For this review, take the finished solid that the model builds, in its own axes (mm). Coordinates: 2 decimals unless noted, no trailing zeros. Loops run counter-clockwise (first coordinate to the right, second up) from the corner with the lowest first, then second, coordinate; pieces in that order, holes last.
1. Mouldability with a two-part tool opening along Y and no side actions: class faces 1 (the face through (2, -20.609, 5)), 2 (the face through (2, 17.491, 2)), 3 (the face through (4.064, -2, 4)), 4 (the face through (2.004, 16.074, 2.901)) as pulls with the +Y half, pulls with the -Y half, needs draft (parallel to the pull), parting line crosses it, or undercut.
2. Clearance check with a flat-ended pin moving along its axis: P1, Ø1.5, axis at x = 2, y = 11.5, coming from the +Z side. State where the tip first meets the part, or that it passes through.
3. Take a section at D-D, the plane y = -8. State the section outline as (x, z) points, then the cut area to 3 significant figures.
4. Take a section at C-C, the plane z = 7.75. State the section outline as (x, y) points.
5. Take a section at B-B, the plane x = 3.45. State the section outline as (y, z) points (3 decimals).
6. To check wall thickness, follow probe 1 along Z at (x, y) = (3.85, 14); probe 2 along Y at (x, z) = (3.45, 4); probe 3 along Y at (x, z) = (1.9, 2). State the ranges of each line that lie inside material, in increasing order.
7. Take a section at A-A, the plane y = -18. State the section outline as (x, z) points.
```python
from build123d import *

# Parameters (mm, degrees)
F1_DEPTH = 4.064
F3_D     = 3.2639
F4_R     = 1.524


with BuildPart() as f1:
    # F0 (on Right) → F1 (new body)
    with BuildSketch(Plane.YZ):
        Polygon((-20.6086377689, 9.525), (-20.6086377689, 0), (17.4913622311, 0), (17.4913622311, 6.35), align=None)
    extrude(amount=F1_DEPTH)

    # F3 (through all)
    with Locations(Plane.YZ.offset(4.064)):
        with Locations((-17.5606377689, 6.8387051621), (14.4433622311, 2.8296108316)):
            Hole(F3_D / 2)

    # F4
    f4_edges = [f1.edges().sort_by_distance(p)[0] for p in [
        (2.032, 17.491362, 6.35),
    ]]
    fillet(f4_edges, radius=F4_R)


solid = f1.part
```
Results list:
1. face 1: pulls with the -Y half
1. face 2: pulls with the +Y half
1. face 3: needs draft
1. face 4: undercut
2. P1: stops at z = 6.91
3. outline: (0, 0) - (4.06, 0) - (4.06, 8.47) - (0, 8.47) - close
3. area: 34.4 mm2
4. outline: (0, -20.61) - (4.06, -20.61) - (4.06, -18.91) - (0, -18.91) - close; (0, -16.21) - (4.06, -16.21) - (4.06, 0.69) - (0, 0.69) - close
5. outline: (-20.609, 0) - (17.491, 0) - (17.491, 4.948) arc R1.524 ccw to (16.094, 6.466) - (-20.609, 9.525) - close; hole circle Ø3.264 at (-17.561, 6.839); hole circle Ø3.264 at (14.443, 2.83)
6. probe 1: z = 0 to 1.26, 4.4 to 6.64
6. probe 2: y = -20.61 to 13.31, 15.58 to 17.49
6. probe 3: y = -20.61 to 13.04, 15.85 to 17.49
7. outline: (0, 0) - (4.06, 0) - (4.06, 5.27) - (0, 5.27) - close; (0, 8.41) - (4.06, 8.41) - (4.06, 9.31) - (0, 9.31) - close
